Verification items for the finished model (mm, model axes). Face numbers are marked on the shaded views. A direction names the side the tool comes from. Coordinates: 2 decimals unless noted, no trailing zeros. Loops run counter-clockwise (first coordinate to the right, second up) from the corner with the lowest first, then second, coordinate; pieces in that order, holes last. Notation, with made-up numbers: (38.25, 81) -> (67.25, 81) arc R23 ccw to (67.25, 119) -> close; hole circle Ø3 at (-4, -7.75). An arc over 180 degrees is marked (long way). Answer as a JSON object with one key per item and string values. Group by question number.
Q1. Release check for a two-part mould opening along Z. For the marked faces 1, 2 and 3 record: released by +Z, released by -Z, zero draft, split by the parting line, or undercut.
Q2. Gauge pin test, flat ends, axial feed: pin 1 Ø12 at (x, z) = (-43.5, -7.5) entering from +Y; pin 2 Ø3.5 at (x, z) = (0, 25.4) entering from +Y; pin 3 Ø3.5 at (x, z) = (-32.99, 9.99) entering from -Y; pin 4 Ø5.5 at (y, z) = (21.59, -18.25) entering from +X. Record the tip position at first contact, or that the pin passes through.
Q3. Cross-section at C-C on y = 71. Record the boundary of the cut face in (x, z), and give its area (3 significant figures).
Q4. Scan lines: L1, parallel to Z at x = -43.65, y = 0.6; L2, parallel to Z at x = 31, y = 34.5; L3, parallel to X at y = 0.9, z = -42.38. Record each from-to range of solid material in increasing order.
Q5. Cross-section at A-A on y = 21.59. Record the boundary of the cut face in (x, z).
Q6. Cross-section at B-B on z = -25.4. Record the boundary of the cut face in (x, y).
Q7. Set-up check for the marked faces 4 and 5: record each of +Z, -Z, +X, -X, +Y, -Y from which the full face is reachable in a straight line by a thin tool's end or side.
Autodesk Inventor part; units mm, degrees
ref_plane "YZ Plane" through (0, 0, 0) normal (1, 0, 0) x (0, 1, 0)
ref_plane "XZ Plane" through (0, 0, 0) normal (0, 1, 0) x (-1, 0, 0)
ref_plane "XY Plane" through (0, 0, 0) normal (0, 0, 1) x (1, 0, 0)
sketch "Sketch1" plane through (0, 0, 0) normal (0, 1, 0) x (-1, 0, 0)
  line L0 (-60.452, -60.452) -> (60.452, -60.452)
  line L1 (60.452, -60.452) -> (60.452, 60.452)
  line L2 (60.452, 60.452) -> (-60.452, 60.452)
  line L3 (-60.452, 60.452) -> (-60.452, -60.452)
  line L4 (-60.452, -60.452) -> (60.452, 60.452) construction
  line L5 (60.452, -60.452) -> (-60.452, 60.452) construction
  point P0 (0, 0)
  dimension "d0" = 120.904
  dimension "d1" = 120.904
extrude "Extrusion1" add sketch "Sketch1" along normal blind 2.54
sketch "Sketch2" plane through (0, 2.54, 0) normal (0, 1, 0) x (1, 0, 0)
  line L0 (60.452, 60.452) -> (-60.452, 60.452)
  line L1 (60.452, -60.452) -> (-60.452, -60.452)
  line L2 (-60.452, -60.452) -> (-60.452, 60.452)
  line L3 (-60.452, 60.452) -> (60.452, 60.452)
  line L4 (60.452, 60.452) -> (60.452, -60.452)
  line L5 (60.452, -60.452) -> (-60.452, 60.452) construction
  line L6 (-60.452, -60.452) -> (60.452, 60.452) construction
  line L7 (59.182, -59.182) -> (-59.182, -59.182)
  line L8 (-59.182, -59.182) -> (-59.182, 59.182)
  line L9 (-59.182, 59.182) -> (59.182, 59.182)
  line L10 (59.182, 59.182) -> (59.182, -59.182)
  line L11 (59.182, -59.182) -> (-59.182, 59.182) construction
  line L12 (-59.182, -59.182) -> (59.182, 59.182) construction
  point P0 (0, 0)
  dimension "d4" = 118.364
  dimension "d5" = 118.364
extrude "Extrusion2" add sketch "Sketch2" along normal blind 82.804
sketch "Sketch3" plane through (0, 2.54, 0) normal (0, 1, 0) x (1, 0, 0)
  circle A0 centre (0, -25.4) radius 2.0828
  circle A1 centre (0, 25.4) radius 2.0828
  point P0 (0, 0)
  dimension "d10" = 4.1656
  dimension "d11" = 4.1656
extrude "Extrusion3" cut sketch "Sketch3" against normal through all
sketch "Sketch4" plane through (0, 2.54, 0) normal (0, 1, 0) x (1, 0, 0)
  line L0 (50, -50) -> (-50, 50) construction
  line L1 (-50, -50) -> (50, 50) construction
  circle A0 centre (41.6656, 7.15) radius 1.4224
  circle A1 centre (-43.65, -42.38) radius 1.4224
  circle A2 centre (-43.65, 42.38) radius 1.4224
  line L2 (32.9946, -9.9949) -> (-32.9946, 9.9949) construction
  line L3 (-32.9946, -9.9949) -> (32.9946, 9.9949) construction
  circle A3 centre (-32.9946, -9.9949) radius 1.4986
  circle A4 centre (-32.9946, 9.9949) radius 1.4986
  circle A5 centre (32.9946, 9.9949) radius 1.4986
  circle A6 centre (32.9946, -9.9949) radius 1.4986
  point P0 (0, 0)
  dimension "d14" = 100
  dimension "d15" = 100
  dimension "d21" = 2.8448
  dimension "d22" = 2.8448
  dimension "d23" = 2.8448
  dimension "d24" = 65.9892
  dimension "d25" = 19.9898
  dimension "d26" = 2.9972
  dimension "d27" = 2.9972
  dimension "d28" = 2.9972
  dimension "d29" = 2.9972
extrude "Extrusion4" cut sketch "Sketch4" against normal through all
sketch "Sketch5" plane through (-59.182, 2.54, 59.182) normal (1, 0, 0) x (0, 0, -1)
  line L0 (0, 0) -> (0, 82.804)
  line L1 (0, 19.05) -> (9.1821, 19.05) construction
  circle A0 centre (59.1821, 19.05) radius 3.175
  point P0 (59.182, -2.54)
  dimension "d35" = 6.35
extrude "Extrusion5" cut sketch "Sketch5" against normal through all
sketch "Sketch6" plane through (59.182, 2.54, -59.182) normal (-1, 0, 0) x (0, 0, 1)
  point P0 (59.182, -2.54)
sketch "Sketch7" plane through (59.182, 2.54, -59.182) normal (-1, 0, 0) x (0, 0, 1)
  line L0 (0, 0) -> (0, 82.804)
  line L1 (0, 19.05) -> (9.1821, 19.05) construction
  circle A0 centre (29.0259, 19.05) radius 3.175
  circle A1 centre (40.9321, 19.05) radius 3.175
  circle A2 centre (75.8571, 19.05) radius 3.175
  circle A3 centre (89.3509, 19.05) radius 3.175
  point P0 (59.182, -2.54)
  dimension "d44" = 6.35
  dimension "d45" = 6.35
  dimension "d46" = 6.35
  dimension "d47" = 6.35
extrude "Extrusion6" cut sketch "Sketch7" against normal through all
properties part number "546-1550Z137-4xSplitter"
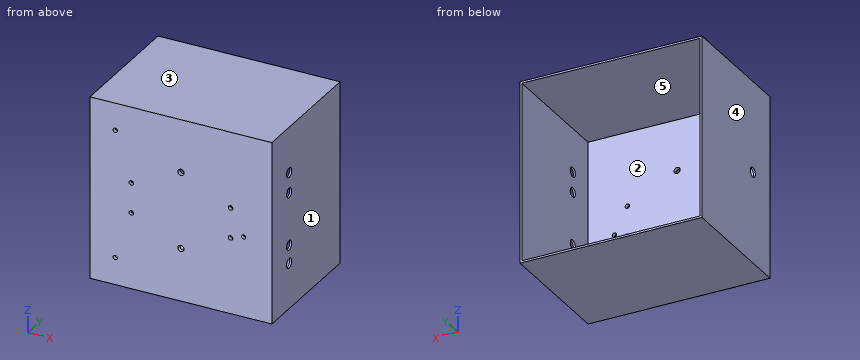
Computed values:
{
 "1": {"face 1": "zero draft", "face 2": "undercut", "face 3": "released by +Z"},
 "2": {"pin 1": "stops at y = 2.54", "pin 2": "passes through", "pin 3": "stops at y = 0", "pin 4": "stops at x = -59.18"},
 "3": {"outline": "(-60.45, -60.45) -> (60.45, -60.45) -> (60.45, 60.45) -> (-60.45, 60.45) -> close; hole (-59.18, -59.18) -> (59.18, -59.18) -> (59.18, 59.18) -> (-59.18, 59.18) -> close", "area": "608 mm²"},
 "4": {"L1": "z = -60.45 to -43.8, -40.96 to 40.96, 43.8 to 60.45", "L2": "z = -60.45 to -59.18, 59.18 to 60.45", "L3": "x = -60.45 to -45.07, -42.23 to 60.45"},
 "5": {"outline": "(-60.45, -60.45) -> (60.45, -60.45) -> (60.45, -33.33) -> (59.18, -33.33) -> (59.18, -59.18) -> (-59.18, -59.18) -> (-59.18, -3.18) -> (-60.45, -3.18) -> close; (-60.45, 3.17) -> (-59.18, 3.17) -> (-59.18, 59.18) -> (59.18, 59.18) -> (59.18, 33.34) -> (60.45, 33.34) -> (60.45, 60.45) -> (-60.45, 60.45) -> close; (59.18, -26.98) -> (60.45, -26.98) -> (60.45, -21.42) -> (59.18, -21.42) -> close; (59.18, -15.07) -> (60.45, -15.07) -> (60.45, 13.5) -> (59.18, 13.5) -> close; (59.18, 19.85) -> (60.45, 19.85) -> (60.45, 26.99) -> (59.18, 26.99) -> close"},
 "6": {"outline": "(-60.45, 0) -> (-2.08, 0) -> (-2.08, 2.54) -> (-59.18, 2.54) -> (-59.18, 85.34) -> (-60.45, 85.34) -> close; (2.08, 0) -> (60.45, 0) -> (60.45, 85.34) -> (59.18, 85.34) -> (59.18, 2.54) -> (2.08, 2.54) -> close"},
 "7": {"face 4": "+Z, -Z, -X, +Y, -Y", "face 5": "+Y"}
}
